Solid Edge part; units mm, degrees
sketch "Sketch1" plane through (0, 117, 0) normal (0, -1, 0) x (1, 0, 0)
  line L0 (-117, 54.9958) -> (-61, 54.9958)
  line L1 (-61, 54.9958) -> (-61, 42.9958)
  line L2 (-61, 42.9958) -> (-20, 42.9958)
  line L3 (-20, 42.9958) -> (-20, 39.4975)
  line L4 (24, 39.4975) -> (-20, 39.4975)
  line L5 (24, 39.4975) -> (24, 36.4958)
  line L6 (24, 36.4958) -> (-117, 36.4958)
  line L7 (-117, 54.9958) -> (-117, 36.4958)
extrude "Protrusion1" add sketch "Sketch1" along normal blind 44
sketch "Sketch2" plane through (-117, 95, 45.2466) normal (-1, 0, 0) x (0, -1, 0)
  line L0 (9, 1.7492) -> (16, 1.7492)
  line L1 (16, 1.7492) -> (16, 6.2492)
  line L2 (16, 6.2492) -> (1, 6.2492)
  line L3 (-14, 6.2492) -> (1, 6.2492)
  line L4 (-14, 1.7492) -> (-14, 6.2492)
  line L5 (-7, 1.7492) -> (-14, 1.7492)
  line L6 (-7, -2.2508) -> (-7, 1.7492)
  line L7 (-7, -2.2508) -> (9, -2.2508)
  line L8 (9, -2.2508) -> (9, 1.7492)
extrude "Cutout1" cut sketch "Sketch2" against normal up to next
sketch "Sketch3" plane through (-2.5, 73, 39.2466) normal (0, -1, 0) x (1, 0, 0)
  line L0 (-17.5, 1.7508) -> (-19, 1.7508)
  line L1 (-19, 1.7508) -> (-19, 0.2508)
  line L2 (-19, 0.2508) -> (-17.5, 0.2508)
  line L3 (-17.5, 0.2508) -> (-17.5, 1.7508)
extrude "Cutout2" cut sketch "Sketch3" against normal up to next
sketch "Sketch4" plane through (3.25, 95, 39.4975) normal (0, 0, 1) x (1, 0, 0)
  line L0 (20.75, -22) -> (20.75, -18)
  line L1 (20.75, -18) -> (-24.25, -18)
  line L2 (-24.25, -18) -> (-28.25, -22)
  line L3 (20.75, -22) -> (-28.25, -22)
extrude "Cutout3" cut sketch "Sketch4" against normal up to next and the other way up to next
sketch "Sketch5" plane through (-46.5, 92.5, 36.4958) normal (0, 0, -1) x (0, 1, 0)
  line L0 (-15.5, 60.5) -> (24.5, 60.5)
  line L1 (24.5, 60.5) -> (24.5, 70.5)
  line L2 (24.5, 70.5) -> (-15.5, 70.5)
  line L3 (-15.5, 70.5) -> (-15.5, 60.5)
extrude "ExtrudedProtrusion_6" add sketch "Sketch5" along normal blind 8
sketch "Sketch6" plane through (24, 98.5, 34.4966) normal (1, 0, 0) x (0, 1, 0)
  line L0 (2.5, -2.5008) -> (2.5, 1.9992)
  line L1 (2.5, 1.9992) -> (-18.5, 1.9992)
  line L2 (-18.5, 1.9992) -> (-18.5, -2.5008)
  line L3 (-18.5, -2.5008) -> (2.5, -2.5008)
extrude "Cutout4" cut sketch "Sketch6" against normal up to next
sketch "Sketch7" plane through (-71, 73, 45.7458) normal (0, -1, 0) x (1, 0, 0)
  line L0 (10, 50.75) -> (10, 9.25)
  line L1 (10, 9.25) -> (-10, 9.25)
  line L2 (-10, 9.25) -> (-10, -9.25)
  line L3 (-10, -9.25) -> (46, -9.25)
  line L4 (46, 50.75) -> (46, -9.25)
  line L5 (10, 50.75) -> (46, 50.75)
extrude "ExtrudedProtrusion_7" add sketch "Sketch7" along normal blind 6
chamfer "Chamfer_4" distance 15 angle 21.5 1 edges at (-81, 67, 45.7458) measured on face at (-52.44, 67, 87.0958)
sketch "Sketch8" plane through (-47.75, 67, 59.9958) normal (0, -1, 0) x (1, 0, 0)
  line L0 (2.25, -17) -> (2.25, 23)
  line L1 (2.25, 23) -> (12.25, 23)
  line L2 (12.25, 23) -> (12.25, -17)
  line L3 (12.25, -17) -> (2.25, -17)
extrude "Cutout5" cut sketch "Sketch8" against normal up to next
sketch "Sketch9" plane through (-47.75, 67, 59.9958) normal (0, -1, 0) x (1, 0, 0)
  line L0 (14.45, -17) -> (0.05, -17)
  line L1 (0.05, 23) -> (0.05, -17)
  line L2 (0.05, 23) -> (14.45, 23)
  line L3 (14.45, 23) -> (14.45, -17)
extrude "ExtrudedCutout_8" cut sketch "Sketch9" against normal blind 1.5
sketch "Sketch10" plane through (-89, 92.5, 54.9958) normal (0, 0, 1) x (0, -1, 0)
  line L0 (25.5, 23) -> (-24.5, 23)
  line L1 (-24.5, 23) -> (-24.5, 28)
  line L2 (-24.5, 28) -> (25.5, 28)
  line L3 (25.5, 28) -> (25.5, 23)
extrude "Protrusion2" add sketch "Sketch10" along normal up to vertex (41.5 mm away)
sketch "Sketch11" plane through (-45.5, 92, 96.4958) normal (0, 0, 1) x (1, 0, 0)
  line L0 (20.5, -20) -> (-15.5, -20)
  line L1 (-15.5, -20) -> (-15.5, -19)
  line L2 (-15.5, -19) -> (20.5, -19)
  line L3 (20.5, -19) -> (20.5, -20)
extrude "Cutout6" cut sketch "Sketch11" against normal up to vertex (53.5 mm away)
CAD build for the part. Positions are in the model's coordinates, mm. A direction names the side the tool comes from. Coordinates: 2 decimals unless noted, no trailing zeros. Write each loop counter-clockwise with the first axis right and the second up, starting at its lowest first coordinate (ties: lowest second). Pieces come first, ordered by that corner, then holes.
(1) Two-plate mould, pull along Y, no slides. Class faces 4 (the face through (-47, 72, 70)), 5 (the face through (-73.605, 69.996, 45.875)), 6 (the face through (19, 90, 31.996)), 7 (the face through (-89, 102, 45)): +Y half, -Y half, draft (parallel to the pull), parting line (faces both ways), or undercut.
(2) Cut at D-D, the plane z = 50. List the corners of the cut face in (x, y).
(3) 3-axis set-ups, long thin cutter, end or side, ignore diameter. For faces 1 (the face through (19, 101, 34)), 2 (the face through (-92, 92, 54.996)), 3 (the face through (-35.5, 70, 63)): which of +Z, -Z, +X, -X, +Y, -Y reach the whole face in a straight line?
(4) Flat gauge pins, fed straight in: pin 1 (3 mm diameter, centred on x = -75.5, z = 45, fed in from -Y); pin 2 (15 mm diameter, centred on x = -97, y = 101, fed in from +Z); pin 3 (1 mm diameter, centred on x = -21, y = 95, fed in from -Z). Where does each tip first touch, or does it go through?
(5) Drill centre lines: probe 1 along Z at (x, y) = (-99, 104.5); probe 2 along Z at (x, y) = (-21, 86); probe 3 along Y at (x, z) = (13, 39). Where is each one in solid material? Low to high.
(6) Cut at C-C, the plane z = 63.5. List the corners of the cut face in (x, y).
(7) Cut at A-A, the plane x = -93.5. List the corners of the cut face in (y, z), and give its area (3 significant figures).
(8) Cut at B-B, the plane y = 82.5. Count the separate pieces of the cut face and the enclosed holes in it, and give its area (3 significant figures).
Geometry says:
1. face 4: +Y half
1. face 5: -Y half
1. face 6: undercut
1. face 7: undercut
2. outline: (-117, 73) - (-81, 73) - (-81, 72.91) - (-66, 67) - (-47.7, 67) - (-47.7, 68.5) - (-45.5, 68.5) - (-45.5, 72) - (-61, 72) - (-61, 79) - (-117, 79) - close; (-117, 109) - (-61, 109) - (-61, 117) - (-117, 117) - close; (-35.5, 68.5) - (-33.3, 68.5) - (-33.3, 67) - (-25, 67) - (-25, 72) - (-35.5, 72) - close
3. face 1: +X, -X
3. face 2: +Z, -X, +Y, -Y
3. face 3: +Y, -Y
4. pin 1: stops at y = 70.15
4. pin 2: stops at z = 55
4. pin 3: stops at z = 36.5
5. probe 1: z = 36.5 to 47, 51.5 to 55
5. probe 2: z = 36.5 to 39.5, 41 to 43
5. probe 3: y = 77 to 117
6. outline: (-66, 67) - (-47.7, 67) - (-47.7, 68.5) - (-45.5, 68.5) - (-45.5, 72) - (-61, 72) - (-61, 117) - (-66, 117) - close; (-35.5, 68.5) - (-33.3, 68.5) - (-33.3, 67) - (-25, 67) - (-25, 72) - (-35.5, 72) - close
7. outline: (73, 36.5) - (117, 36.5) - (117, 55) - (73, 55) - close; hole (79, 47) - (86, 47) - (86, 43) - (102, 43) - (102, 47) - (109, 47) - (109, 51.5) - (79, 51.5) - close
7. area: 615 mm2
8. separate pieces: 3
8. enclosed holes: 0
8. area: 1,420 mm2
